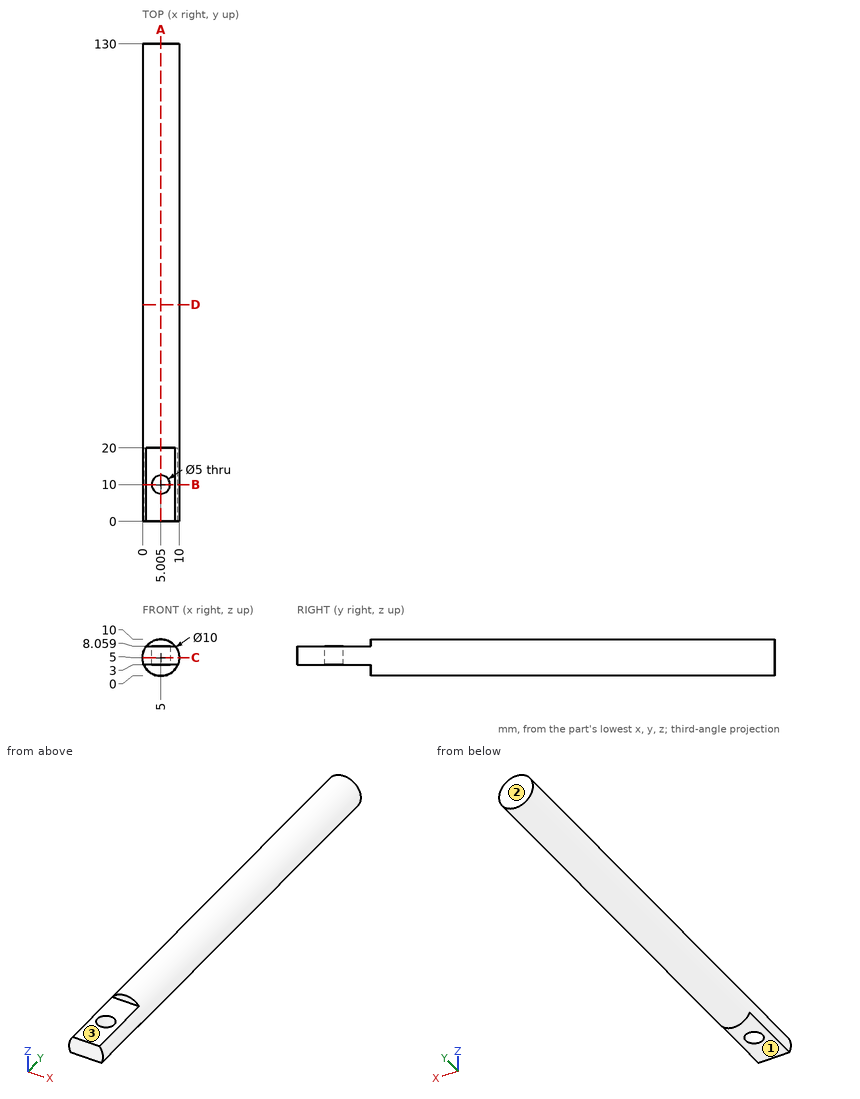
Geometry check sheet. Reference: drawing and pictorial views, mm from the part's lowest x, y, z. A direction names the side the tool comes from. Coordinates: 2 decimals unless noted, no trailing zeros. Order: outer loops, then holes, each group sorted by start corner. A loop starts at its lowest first (then second) coordinate and runs counter-clockwise, first axis right, second up.
Item 1: Depth check by flat-ended pin: pin 1 (1 mm diameter, centred on y = 103, z = 2.5, fed in from -X); pin 2 (6 mm diameter, centred on x = 3, y = 31, fed in from -Z); pin 3 (2 mm diameter, centred on y = 101, z = 3, fed in from +X); pin 4 (0.6 mm diameter, centred on x = 3.5, z = 9, fed in from -Y). Enter the tip coordinate at first touch or a pass-through.
Filled in:
pin 1: stops at x = 0.42
pin 2: stops at z = 0
pin 3: stops at x = 9.9
pin 4: stops at y = 20
Item 2: Section check B-B, the plane y = 10. Enter the section's corners in (x, z) (1 decimal), then the cut area to 3 significant figures.
Filled in:
outline: (0.4, 3) - (2.5, 3) - (2.5, 8.1) - (1, 8.1) arc R5 ccw to start; (7.5, 3) - (9.6, 3) arc R5 ccw to (9, 8.1) - (7.5, 8.1) - close
area: 22.7 mm2
Item 3: Section check C-C, the plane z = 5. Enter the section's corners in (x, y) (3 decimals), then the cut area to 3 significant figures.
Filled in:
outline: (0, 0) - (10, 0) - (10, 130) - (0, 130) - close; hole circle Ø5 at (5.005, 10)
area: 1,280 mm2
Item 4: Material ranges on L1, parallel to Z at x = 3, y = 43; L2, parallel to Y at x = 2, z = 8.5; L3, parallel to Z at x = 2, y = 18, recorded low to high.
Filled in:
L1: z = 0.42 to 9.58
L2: y = 20 to 130
L3: z = 3 to 8.06
Item 5: Section check A-A, the plane x = 5. Enter the section's corners in (y, z), then the cut area to 3 significant figures.
Filled in:
outline: (0, 3) - (7.5, 3) - (7.5, 8.06) - (0, 8.06) - close; (12.5, 3) - (20, 3) - (20, 0) - (130, 0) - (130, 10) - (20, 10) - (20, 8.06) - (12.5, 8.06) - close
area: 1,180 mm2
Item 6: Access from +Z, -Z, +X, -X, +Y, -Y to the whole of each face (thin tool, end or side, straight path). Record for the marked faces 1, 2 and 3.
Filled in:
face 1: -Z, +X, -X, -Y
face 2: +Z, -Z, +X, -X, +Y
face 3: +Z, +X, -X, -Y
Item 7: Section check D-D, the plane y = 59. Enter the section's corners in (x, z).
Filled in:
outline: circle Ø10 at (5, 5)
